Autodesk Inventor part; units mm, degrees
ref_plane "YZ Plane" through (0, 0, 0) normal (1, 0, 0) x (0, 1, 0)
ref_plane "XZ Plane" through (0, 0, 0) normal (0, 1, 0) x (-1, 0, 0)
ref_plane "XY Plane" through (0, 0, 0) normal (0, 0, 1) x (1, 0, 0)
sketch "Sketch1" plane through (0, 0, 0) normal (0, 0, 1) x (1, 0, 0)
  arc A0 (-25.4018, 15) -> (25.4018, 15) centre (0, 0) ccw
  line L0 (-39, 2.5) -> (-32, 2.5)
  line L1 (-32, -2.5) -> (-39, -2.5)
  line L2 (-39, -2.5) -> (-39, 2.5)
  line L3 (-32, 2.5) -> (-31.9022, 2.5)
  line L4 (-32, -2.5) -> (-31.9022, -2.5)
  line L5 (2.5, -32) -> (2.5, -39)
  line L6 (2.5, -39) -> (-2.5, -39)
  line L7 (-2.5, -39) -> (-2.5, -32)
  line L8 (-2.5, -32) -> (-2.5, -31.9022)
  line L9 (2.5, -32) -> (2.5, -31.9022)
  line L10 (32, 2.5) -> (31.9022, 2.5)
  line L11 (32, -2.5) -> (31.9022, -2.5)
  arc A1 (-28.2666, 15) -> (-31.9022, 2.5) centre (0, 0) ccw
  arc A2 (-31.9022, -2.5) -> (-2.5, -31.9022) centre (0, 0) ccw
  arc A3 (2.5, -31.9022) -> (31.9022, -2.5) centre (0, 0) ccw
  arc A4 (31.9022, 2.5) -> (28.2666, 15) centre (0, 0) ccw
  arc A5 (12.5, 26.7208) -> (25.4018, 15) centre (0, 0) ccw
  line L12 (12.5, 29.4576) -> (12.5, 26.7208)
  arc A6 (-2.5, 31.9022) -> (-31.9022, 2.5) centre (0, 0) ccw
  arc A7 (-31.9022, -2.5) -> (-2.5, -31.9022) centre (0, 0) ccw
  arc A8 (2.5, -31.9022) -> (31.9022, -2.5) centre (0, 0) ccw
  arc A9 (31.9022, 2.5) -> (28.2666, 15) centre (0, 0) ccw
  line L13 (6.5, 31.3329) -> (7.5001, 38.3601)
  line L14 (6.5, 31.3329) -> (13.598, 31.3329) construction
  line L15 (7.5001, 38.3601) -> (12.4502, 37.6556)
  line L16 (12.4502, 37.6556) -> (11.3493, 29.9198)
  arc A10 (12.5, 29.4576) -> (11.3493, 29.9198) centre (0, 0) ccw
  arc A11 (12.5, 29.4576) -> (11.3493, 29.9198) centre (0, 0) ccw
  arc A12 (6.5, 31.3329) -> (2.5, 31.9022) centre (0, 0) ccw
  arc A13 (6.5, 31.3329) -> (-31.9022, 2.5) centre (0, 0) ccw
  arc A14 (31.9022, 2.5) -> (28.2666, 15) centre (0, 0) ccw
  arc A15 (-31.9022, -2.5) -> (-2.5, -31.9022) centre (0, 0) ccw
  arc A16 (2.5, -31.9022) -> (31.9022, -2.5) centre (0, 0) ccw
  line L17 (31.9022, 2.5) -> (41.0332, 2.5) construction
  line L18 (29.8114, 11.631) -> (36.8386, 12.6311)
  line L19 (29.8114, 11.631) -> (36.9094, 11.631) construction
  line L20 (36.8386, 12.6311) -> (41.8386, 12.6311) construction
  line L21 (36.8386, 12.6311) -> (36.1341, 17.5812)
  line L22 (36.8386, 12.6311) -> (41.8386, 12.6311) construction
  line L23 (36.1341, 17.5812) -> (27.5058, 16.3533)
  line L24 (36.1341, 17.5812) -> (44.8493, 17.5812) construction
  arc A17 (12.5, 26.7208) -> (24.5524, 16.3533) centre (0, 0) ccw
  arc A18 (12.5, 29.4576) -> (11.3493, 29.9198) centre (0, 0) ccw
  arc A19 (2.5, -31.9022) -> (27.5058, 16.3533) centre (0, 0) ccw
  arc A20 (6.5, 31.3329) -> (-31.9022, 2.5) centre (0, 0) ccw
  arc A21 (-31.9022, -2.5) -> (-2.5, -31.9022) centre (0, 0) ccw
  arc A22 (12.5, 26.7208) -> (22.9783, 18.5) centre (0, 0) ccw
  line L25 (28.2666, 15) -> (31.7666, 15) construction
  line L26 (22.9783, 18.5) -> (26.1103, 18.5)
  arc A23 (12.5, 29.4576) -> (11.3493, 29.9198) centre (0, 0) ccw
  arc A24 (6.5, 31.3329) -> (-31.9022, 2.5) centre (0, 0) ccw
  arc A25 (-31.9022, -2.5) -> (-2.5, -31.9022) centre (0, 0) ccw
  arc A26 (2.5, -31.9022) -> (26.1103, 18.5) centre (0, 0) ccw
  point P0 (11.5, 29.8622)
  point P1 (2.5, 31.9022)
  point P2 (24.5524, 16.3533)
  point P3 (25.4018, 15)
  dimension "d78" = 7.098
  dimension "d79" = 81.9
  dimension "d80" = 5
  dimension "d81" = 90
  dimension "d82" = 90
  dimension "d89" = 7.098
  dimension "d90" = 8.1
  dimension "d93" = 5
  dimension "d94" = 98.1
  dimension "d95" = 171.9
extrude "Extrusion7" add sketch "Sketch1" along normal blind 5
properties part number "Clip_TestFitV1"
Verification items for the finished model (mm, model axes). A direction names the side the tool comes from. Round coordinates to 2 decimals unless told otherwise and drop trailing zeros. Order: outer loops, then holes, each group sorted by start corner. A loop starts at its lowest first (then second) coordinate and runs counter-clockwise, first axis right, second up.
1) Cross-section at C-C, the plane z = 2.65. Record the cut outline in (x, y), plus the area to 3 significant figures.
Geometry says:
outline: (-39, -2.5) - (-31.9, -2.5) arc R32 ccw to (-2.5, -31.9) - (-2.5, -39) - (2.5, -39) - (2.5, -31.9) arc R32 ccw to (31.9, -2.5) arc R32 ccw to (31.9, 2.5) arc R32 ccw to (29.81, 11.63) - (36.84, 12.63) - (36.13, 17.58) - (27.51, 16.35) arc R32 ccw to (26.11, 18.5) - (22.98, 18.5) arc R29.5 cw to (24.55, 16.35) arc R29.5 cw to (25.4, 15) arc R29.5 cw (long way) to (-25.4, 15) arc R29.5 cw to (12.5, 26.72) - (12.5, 29.46) arc R32.04 ccw to (11.35, 29.92) - (12.45, 37.66) - (7.5, 38.36) - (6.5, 31.33) arc R32 ccw to (2.5, 31.9) arc R32 ccw to (-2.5, 31.9) arc R32 ccw to (-28.27, 15) arc R32 ccw to (-31.9, 2.5) - (-39, 2.5) - close
area: 591 mm2
2) Draft check along X on faces 1 (the cylindrical face through (-30.75, 8.85, 2.46)), 2 (the flat face through (7, -29, 5)), 3 (the cylindrical face through (26.82, 17.456, 2.465)). Enter one of: +X half, -X half, draft (parallel to the pull), parting line (faces both ways), or undercut.
Geometry says:
face 1: -X half
face 2: draft
face 3: undercut
3) Depth check by flat-ended pin: pin 1 (0.8 mm diameter, centred on y = 28.5, z = 2, fed in from +X); pin 2 (1.6 mm diameter, centred on x = 25, z = 1.5, fed in from +Y); pin 3 (1.5 mm diameter, centred on x = -37, z = 3, fed in from +Y). Enter the tip coordinate at first touch or a pass-through.
Geometry says:
pin 1: stops at x = 12.5
pin 2: stops at y = 18.5
pin 3: stops at y = 2.5
4) Cross-section at D-D, the plane x = 20.5. Record the cut outline in (y, z).
Geometry says:
outline: (-24.57, 0) - (-21.21, 0) - (-21.21, 5) - (-24.57, 5) - close
5) Tool access check on faces 4 (the flat face through (12.5, 28, 2)), 5 (the flat face through (11.9, 33.8, 2.5)), 6 (the flat face through (-2.5, -36, 2)). Record the directions out of +Z, -Z, +X, -X, +Y, -Y that give a thin tool (end or side, any length) a straight path to the whole face; none if there is none.
Geometry says:
face 4: +Z, -Z, +X, +Y
face 5: +Z, -Z, +X
face 6: +Z, -Z, -X, -Y
6) Cross-section at A-A, the plane y = 0. Record the cut outline in (x, z).
Geometry says:
outline: (-39, 0) - (-29.5, 0) - (-29.5, 5) - (-39, 5) - close; (29.5, 0) - (32, 0) - (32, 5) - (29.5, 5) - close
7) Material ranges on line 1 (Y direction, x = 0, z = 3.45); line 2 (Y direction, x = -32.5, z = 1.45), recorded low to high.
Geometry says:
line 1: y = -39 to -29.5, 29.5 to 32
line 2: y = -2.5 to 2.5
